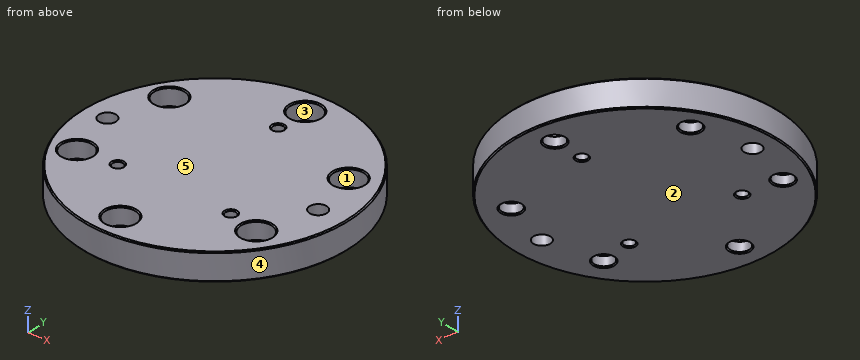
```python
from build123d import *

# Parameters (mm, degrees)
F0_R           = 62
F1_DEPTH       = 12.7
F2_D           = 5
F4_D           = 9
F4_CBORE_D     = 14.25
F4_CBORE_DEPTH = 8
F5_SIZE        = 0.5
F6_D           = 8


# Not quite as in the source:
# - a feature names something its author has since deleted; it is built from what else it names


with BuildPart() as f1:
    # F0 (on Top) → F1 (new body)
    with BuildSketch(Plane.XY):
        Circle(F0_R)
    extrude(amount=F1_DEPTH)

    # F2 (through all)
    with Locations(Plane(origin=(0, 0, 0), x_dir=(1, 0, 0), z_dir=(0, 0, -1))):
        with Locations((0, -35), (26.8, 22.5), (-26.8, 22.5)):
            Hole(F2_D / 2)

    # F4 (through all)
    with Locations(Plane.XY.offset(12.7)):
        with Locations((0, 50), (-43.8068557852, 25.8756999398), (42.7956845933, 24.1243000602), (-44.8180269771, -24.1243000602), (-2.0223423839, -50), (41.7845134013, -25.8756999398)):
            CounterBoreHole(F4_D / 2, F4_CBORE_D / 2, F4_CBORE_DEPTH)

    # F5
    f5_edges = [f1.edges().sort_by_distance(p)[0] for p in [
        (-62, 0, 12.7),
        (-9.147342, -50, 12.7),
        (-51.943027, -24.1243, 12.7),
        (-29.3, -22.5, 12.7),
        (24.3, -22.5, 12.7),
        (34.659513, -25.8757, 12.7),
        (-50.931856, 25.8757, 12.7),
        (35.670685, 24.1243, 12.7),
        (-2.5, 35, 12.7),
        (-7.125, 50, 12.7),
        (-62, 0, 0),
        (-6.522342, -50, 0),
        (-49.318027, -24.1243, 0),
        (-29.3, -22.5, 0),
        (24.3, -22.5, 0),
        (37.284513, -25.8757, 0),
        (-48.306856, 25.8757, 0),
        (38.295685, 24.1243, 0),
        (-2.5, 35, 0),
        (-4.5, 50, 0),
    ]]
    chamfer(f5_edges, length=F5_SIZE)

    # F6 (through all)
    with Locations(Plane.XY.offset(12.7)):
        with Locations((-51.0111711919, 0), (48.9888288081, 0)):
            Hole(F6_D / 2)


solid = f1.part
```
For this review, take the finished solid that the model builds, in its own axes (mm). Face numbers are marked on the shaded views. A direction names the side the tool comes from. Round coordinates to 2 decimals unless told otherwise and drop trailing zeros. Use CSV: the item, a comma, the result in double quotes.
1) Clearance check with flat-ended pins moving along their axes: pin 1 Ø1.5 at (x, z) = (-41.5, 4.5) entering from +Y; pin 2 Ø7 at (x, y) = (41.78, -25.88) entering from -Z; pin 3 Ø18.5 at (x, y) = (-44.82, -24.12) entering from +Z; pin 4 Ø11.5 at (x, y) = (-43.81, 25.88) entering from +Z. State where each tip first meets the part, or that it passes through.
Conclusion:
pin 1,"stops at y = 46.73"
pin 2,"passes through"
pin 3,"stops at z = 12.7"
pin 4,"stops at z = 4.7"
2) For the marked faces 1 and 2, list the 3-axis set-ups (+Z, -Z, +X, -X, +Y, -Y) from which the entire face can be reached by the end or side of a thin tool; tool diameter is ignored.
Conclusion:
face 1,"+Z"
face 2,"-Z, +X, -X, +Y, -Y"
3) The part is to be moulded in two halves that separate along X. For the marked faces 3, 4 and 5, say which applies: pulls with the +X half, pulls with the -X half, needs draft (parallel to the pull), parting line crosses it, or undercut.
Conclusion:
face 3,"undercut"
face 4,"parting line crosses it"
face 5,"needs draft"
4) Wall thickness on line 1 along Y through (x, z) = (0, 12) (3 decimals); line 2 along X through (y, z) = (-3.5, 10.5); line 3 along Y through (x, z) = (38.5, 4.75): over which ranges is each line inside the solid? List them lowest first. Write a range as from..to.
Conclusion:
line 1,"y = -62..-56.832, -43.168..32.5, 37.5..42.875, 57.125..62"
line 2,"x = -61.9..-52.95, -49.07..47.05, 50.93..61.9"
line 3,"y = -48.6..-32.2, -19.55..18.44, 29.81..48.6"
5) Add section A-A on z = 7.75. Count the separate pieces of the cut face and the enclosed holes in it, and give its area (3 significant figures).
Conclusion:
separate pieces,"1"
enclosed holes,"11"
area,"11,000 mm^2"
